The model under review builds one solid part; all positions refer to its coordinate system, in mm. Face numbers are marked on the shaded views. A direction names the side the tool comes from. Give positions to 0.01 mm unless a question says otherwise; leave off trailing zeros. Write each loop counter-clockwise with the first axis right and the second up, starting at its lowest first coordinate (ties: lowest second). Pieces come first, ordered by that corner, then holes. Notation, with made-up numbers: M 6.5,34.25 L 21.5,34.25 A8 ccw 21.5,39.25 Z; hole C -19.75,-38.5 d11. An arc over 180 degrees is marked long. Write item = value, one per line. Start each with the question number.
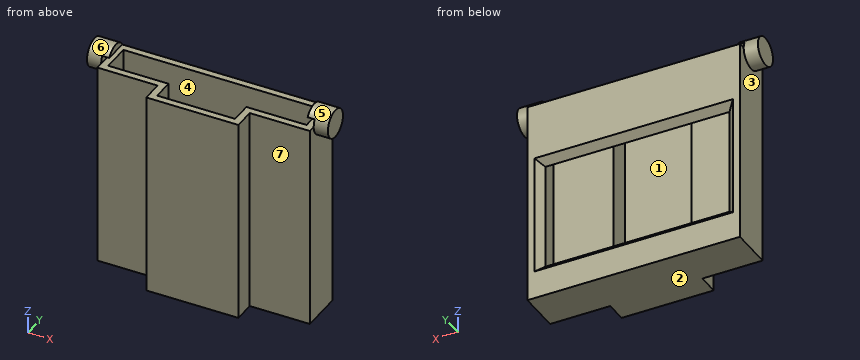
```python
from build123d import *

# Parameters (mm, degrees)
ESQUISSE1_W             = 30
ESQUISSE1_H             = 29
BOSS_EXTRU_1_DEPTH      = 6
COQUE1_T                = -1
ENL_V_MAT_EXTRU_1_REACH = 44.154
ESQUISSE2_W             = 26
ESQUISSE2_H             = 15
ESQUISSE3_W             = 13
ESQUISSE3_H             = 29
BOSS_EXTRU_2_DEPTH      = 3
ESQUISSE5_W             = 11
ESQUISSE5_H             = 28
ENL_V_MAT_EXTRU_2_DEPTH = 3
BOSS_EXTRU_3_DEPTH      = 2
BOSS_EXTRU_3_DEPTH_BACK = 1
ESQUISSE6_R             = 2
BOSS_EXTRU_4_DEPTH      = 2
BOSS_EXTRU_4_DEPTH_BACK = 1
ESQUISSE7_R             = 2
CHANFREIN1_SIZE         = 1
ESQUISSE11_W            = 1
ESQUISSE11_H            = 5.866928615
ENL_V_MAT_EXTRU_5_DEPTH = 1
ESQUISSE12_W            = 1
ESQUISSE12_H            = 9.243044447
ENL_V_MAT_EXTRU_6_DEPTH = 1


with BuildPart() as part:
    # Esquisse1 → Boss.-Extru.1 (new body)
    with BuildSketch(Plane(origin=(0, 0, 0), x_dir=(1, 0, 0), z_dir=(0, 1, 0))):
        with Locations((15, 14.5)):
            Rectangle(ESQUISSE1_W, ESQUISSE1_H)
    extrude(amount=BOSS_EXTRU_1_DEPTH)

    # Coque1
    coque1_openings = [part.faces().sort_by_distance(p)[0] for p in [
        (15, 3, 0),
    ]]
    offset(amount=COQUE1_T, openings=coque1_openings, kind=Kind.INTERSECTION)

    # Esquisse2 → Enlèv. mat.-Extru.1 (cut, up to next)
    with BuildSketch(Plane(origin=(0, 6, 0), x_dir=(1, 0, 0), z_dir=(0, 1, 0)), mode=Mode.PRIVATE) as enl_v_mat_extru_1_sk1:
        with Locations((15, 16.5)):
            Rectangle(ESQUISSE2_W, ESQUISSE2_H)
    enl_v_mat_extru_1_tool1 = extrude(enl_v_mat_extru_1_sk1.sketch, amount=-ENL_V_MAT_EXTRU_1_REACH, mode=Mode.PRIVATE) & part.part
    add(enl_v_mat_extru_1_tool1.solids().sort_by_distance((15, 6, -16.5))[0], mode=Mode.SUBTRACT)

    # Esquisse3 → Boss.-Extru.2 (add)
    with BuildSketch(Plane.XZ):
        with Locations((15, -14.5)):
            Rectangle(ESQUISSE3_W, ESQUISSE3_H)
    extrude(amount=BOSS_EXTRU_2_DEPTH)

    # Esquisse5 → Enlèv. mat.-Extru.2 (cut)
    with BuildSketch(Plane(origin=(0, 1, 0), x_dir=(1, 0, 0), z_dir=(0, 1, 0))):
        with Locations((15, 14)):
            Rectangle(ESQUISSE5_W, ESQUISSE5_H)
    extrude(amount=-ENL_V_MAT_EXTRU_2_DEPTH, mode=Mode.SUBTRACT)

    # Esquisse6 → Boss.-Extru.3 (add, two sides: drawn at the far end of the back side and taken through both)
    with BuildSketch(Plane(origin=(30, 0, 0), x_dir=(0, 0, -1), z_dir=(1, 0, 0)).offset(-BOSS_EXTRU_3_DEPTH_BACK)):
        with Locations((0, 3)):
            Circle(ESQUISSE6_R)
    extrude(amount=BOSS_EXTRU_3_DEPTH + BOSS_EXTRU_3_DEPTH_BACK)

    # Esquisse7 → Boss.-Extru.4 (add, two sides: drawn at the far end of the back side and taken through both)
    with BuildSketch(Plane.ZY.offset(-BOSS_EXTRU_4_DEPTH_BACK)):
        with Locations(Location((0, 3, 0), (0, 0, 180))):
            Circle(ESQUISSE7_R)
    extrude(amount=BOSS_EXTRU_4_DEPTH + BOSS_EXTRU_4_DEPTH_BACK)

    # Chanfrein1
    chanfrein1_edges = [part.edges().sort_by_distance(p)[0] for p in [
        (15, 6, -24),
        (28, 6, -16.5),
        (15, 6, -9),
        (2, 6, -16.5),
    ]]
    chamfer(chanfrein1_edges, length=CHANFREIN1_SIZE - 0.0001)  # a hair under: the kernel refuses the full size

    # Esquisse11 → Enlèv. mat.-Extru.5 (cut)
    with BuildSketch(Plane.ZY.offset(-29)):
        with Locations((0.5, 3.436697282)):
            Rectangle(ESQUISSE11_W, ESQUISSE11_H)
    extrude(amount=-ENL_V_MAT_EXTRU_5_DEPTH, mode=Mode.SUBTRACT)

    # Esquisse12 → Enlèv. mat.-Extru.6 (cut)
    with BuildSketch(Plane(origin=(1, 0, 0), x_dir=(0, 0, -1), z_dir=(1, 0, 0))):
        with Locations((-0.5, 2.795315934)):
            Rectangle(ESQUISSE12_W, ESQUISSE12_H)
    extrude(amount=-ENL_V_MAT_EXTRU_6_DEPTH, mode=Mode.SUBTRACT)


solid = part.part
```
Item 1: Clearance check with flat-ended pins moving along their axes: P1, Ø3.5, axis at y = -0.5, z = -17, coming from the +X side; P2, Ø2, axis at y = 3.5, z = -20, coming from the -X side; P3, Ø1.5, axis at x = 6.5, z = -10.5, coming from the -Y side. State where each tip first meets the part, or that it passes through.
Item 2: To check wall thickness, follow probe 1 along X at (y, z) = (4.75, -14); probe 2 along X at (y, z) = (-0.75, -12.5); probe 3 along Y at (x, z) = (9, -26.5). State the ranges of each line that lie inside material, in increasing order. Write a range as [from, to].
Item 3: We need section A-A, the plane y = -1. Write out the cut boundary in (x, z).
Item 4: We need section C-C, the plane z = -4. Write out the cut boundary in (x, y).
Item 5: The part is to be moulded in two halves that separate along X. For the marked faces 1, 2 and 3, say which applies: released by +X, released by -X, zero draft, split by the parting line, or undercut.
Item 6: For the marked faces 4, 5, 6 and 7, list the 3-axis set-ups (+Z, -Z, +X, -X, +Y, -Y) from which the entire face can be reached by the end or side of a thin tool; tool diameter is ignored.
Worked out:
q1.P1 = 30
q1.P2 = 0
q1.P3 = 0
q2.probe_1 = [0, 1], [29, 30]
q2.probe_2 = [8.5, 9.5], [20.5, 21.5]
q2.probe_3 = [-3, 1], [5, 6]
q3.outline = M 8.5,-29 L 21.5,-29 L 21.5,0 L 20.5,0 L 20.5,-28 L 9.5,-28 L 9.5,0 L 8.5,0 Z
q4.outline = M 0,0 L 8.5,0 L 8.5,-3 L 21.5,-3 L 21.5,0 L 30,0 L 30,6 L 0,6 Z; hole M 1,1 L 9.5,1 L 9.5,-2 L 20.5,-2 L 20.5,1 L 29,1 L 29,5 L 1,5 Z
q5.face_1 = undercut
q5.face_2 = zero draft
q5.face_3 = released by -X
q6.face_4 = +Z
q6.face_5 = +X
q6.face_6 = -X
q6.face_7 = +Z, -Z, +X, -Y
